Study the drawing (mm; zero at the part's minimum x, y, z) and answer. Give positions to 0.01 mm unless a question says otherwise; leave off trailing zeros. Write each loop counter-clockwise with the first axis right and the second up, starting at its lowest first coordinate (ties: lowest second). Pieces come first, ordered by that corner, then holes. Notation, with made-up numbers: (62, 13) - (67, 13) arc R20 cw to (67, 49) - close; hole circle Ø6 at (50, 78). An arc over 180 degrees is marked (long way). Answer as CSV lines item,"result".
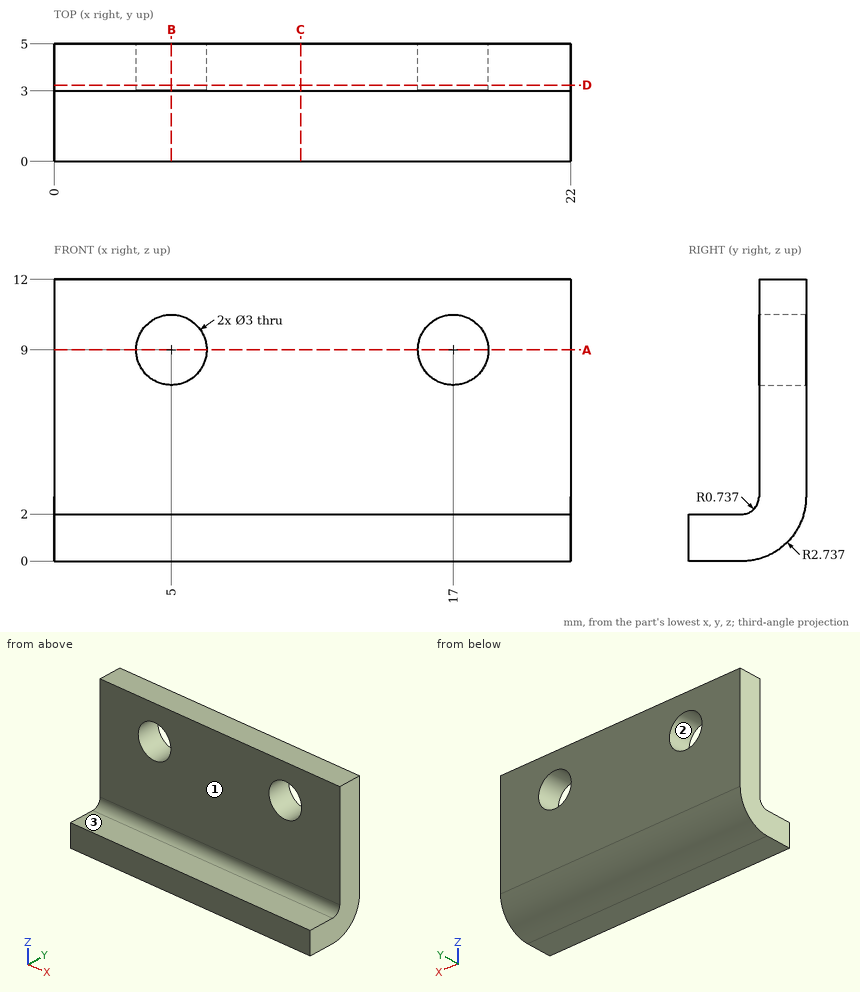
(1) A cutting plane is placed at C-C (x = 10.5). Write down the section's boundary in (y, z).
Worked out:
outline,"(0, 0) - (2.26, 0) arc R2.74 ccw to (5, 2.74) - (5, 12) - (3, 12) - (3, 2.74) arc R0.74 cw to (2.26, 2) - (0, 2) - close"
(2) A cutting plane is placed at A-A (z = 9). Write down the section's boundary in (x, y), and give its area (3 significant figures).
Worked out:
outline,"(0, 3) - (3.5, 3) - (3.5, 5) - (0, 5) - close; (6.5, 3) - (15.5, 3) - (15.5, 5) - (6.5, 5) - close; (18.5, 3) - (22, 3) - (22, 5) - (18.5, 5) - close"
area,"32.0 mm^2"
(3) The mould has two halves that part along Z. Classify the marked faces 1, 2 and 3: +Z half, -Z half, draft (parallel to the pull), parting line (faces both ways), or undercut.
Worked out:
face 1,"draft"
face 2,"undercut"
face 3,"+Z half"
(4) A cutting plane is placed at B-B (x = 5). Write down the section's boundary in (y, z).
Worked out:
outline,"(0, 0) - (2.26, 0) arc R2.74 ccw to (5, 2.74) - (5, 7.5) - (3, 7.5) - (3, 2.74) arc R0.74 cw to (2.26, 2) - (0, 2) - close; (3, 10.5) - (5, 10.5) - (5, 12) - (3, 12) - close"
(5) A cutting plane is placed at D-D (y = 3.25). Write down the section's boundary in (x, z).
Worked out:
outline,"(0, 0.18) - (22, 0.18) - (22, 12) - (0, 12) - close; hole circle Ø3 at (5, 9); hole circle Ø3 at (17, 9)"
(6) Each of these flat-tipped pins is pushed along its axis until it touches: P1, Ø3, axis at x = 16, z = 7, coming from the -Y side; P2, Ø1, axis at y = 1.5, z = 6.5, coming from the +X side; P3, Ø1.1, axis at x = 14.5, y = 0.5, coming from the +Z side. Where does it stop, or does it pass through?
Worked out:
P1,"stops at y = 3"
P2,"passes through"
P3,"stops at z = 2"
(7) Find the intervals of material crossed by L1, parallel to X at y = 4.1, z = 9; L2, parallel to Y at x = 1.25, z = 11; L3, parallel to Z at x = 16.5, y = 0.25, in increasing order.
Worked out:
L1,"x = 0 to 3.5, 6.5 to 15.5, 18.5 to 22"
L2,"y = 3 to 5"
L3,"z = 0 to 2"
